from build123d import *

# Parameters (mm, degrees)
BOSS_EXTRUDE1_DEPTH = 6
CUT_EXTRUDE1_DEPTH  = 6


with BuildPart() as part:
    # Sketch1 → Boss-Extrude1 (new body)
    with BuildSketch(Plane.XY):
        with BuildLine():
            Line((20, 0), (260, 0))
            ThreePointArc((260, 0), (274.142135624, 5.857864376), (280, 20))
            Line((280, 20), (280, 140))
            ThreePointArc((280, 140), (274.142135624, 154.142135624), (260, 160))
            Line((260, 160), (20, 160))
            ThreePointArc((20, 160), (5.857864376, 154.142135624), (0, 140))
            Line((0, 140), (0, 20))
            ThreePointArc((0, 20), (5.857864376, 5.857864376), (20, 0))
        make_face()
    extrude(amount=BOSS_EXTRUDE1_DEPTH)

    # Sketch2 → Cut-Extrude1 (cut)
    with BuildSketch(Plane.XY.offset(6)):
        with BuildLine():
            Line((20, 137.5), (45, 137.5))
            Line((45, 137.5), (45, 122))
            ThreePointArc((45, 122), (47.784318939, 121.672513356), (50.416666667, 120.707928008))
            ThreePointArc((50.416666667, 120.707928008), (53.049014395, 121.672513356), (55.833333333, 122))
            Line((55.833333333, 122), (55.833333333, 137.5))
            Line((55.833333333, 137.5), (80.833333333, 137.5))
            Line((80.833333333, 137.5), (80.833333333, 122))
            ThreePointArc((80.833333333, 122), (83.617652272, 121.672513356), (86.25, 120.707928008))
            ThreePointArc((86.25, 120.707928008), (88.882347728, 121.672513356), (91.666666667, 122))
            Line((91.666666667, 122), (91.666666667, 137.5))
            Line((91.666666667, 137.5), (116.666666667, 137.5))
            Line((116.666666667, 137.5), (116.666666667, 122))
            ThreePointArc((116.666666667, 122), (119.450985605, 121.672513356), (122.083333333, 120.707928008))
            ThreePointArc((122.083333333, 120.707928008), (124.715681061, 121.672513356), (127.5, 122))
            Line((127.5, 122), (127.5, 137.5))
            Line((127.5, 137.5), (152.5, 137.5))
            Line((152.5, 137.5), (152.5, 122))
            ThreePointArc((152.5, 122), (155.284318939, 121.672513356), (157.916666667, 120.707928008))
            ThreePointArc((157.916666667, 120.707928008), (160.549014395, 121.672513356), (163.333333333, 122))
            Line((163.333333333, 122), (163.333333333, 137.5))
            Line((163.333333333, 137.5), (188.333333333, 137.5))
            Line((188.333333333, 137.5), (188.333333333, 122))
            ThreePointArc((188.333333333, 122), (191.117652272, 121.672513356), (193.75, 120.707928008))
            ThreePointArc((193.75, 120.707928008), (196.382347728, 121.672513356), (199.166666667, 122))
            Line((199.166666667, 122), (199.166666667, 137.5))
            Line((199.166666667, 137.5), (224.166666667, 137.5))
            Line((224.166666667, 137.5), (224.166666667, 122))
            ThreePointArc((224.166666667, 122), (226.950985605, 121.672513356), (229.583333333, 120.707928008))
            ThreePointArc((229.583333333, 120.707928008), (232.215681061, 121.672513356), (235, 122))
            Line((235, 122), (235, 137.5))
            Line((235, 137.5), (260, 137.5))
            Line((260, 137.5), (260, 122))
            ThreePointArc((260, 122), (272, 110), (260, 98))
            Line((260, 98), (260, 22.5))
            Line((260, 22.5), (235, 22.5))
            Line((235, 22.5), (235, 98))
            ThreePointArc((235, 98), (232.215681061, 98.327486644), (229.583333333, 99.292071992))
            ThreePointArc((229.583333333, 99.292071992), (226.950985605, 98.327486644), (224.166666667, 98))
            Line((224.166666667, 98), (224.166666667, 22.5))
            Line((224.166666667, 22.5), (199.166666667, 22.5))
            Line((199.166666667, 22.5), (199.166666667, 98))
            ThreePointArc((199.166666667, 98), (196.382347728, 98.327486644), (193.75, 99.292071992))
            ThreePointArc((193.75, 99.292071992), (191.117652272, 98.327486644), (188.333333333, 98))
            Line((188.333333333, 98), (188.333333333, 22.5))
            Line((188.333333333, 22.5), (163.333333333, 22.5))
            Line((163.333333333, 22.5), (163.333333333, 98))
            ThreePointArc((163.333333333, 98), (160.549014395, 98.327486644), (157.916666667, 99.292071992))
            ThreePointArc((157.916666667, 99.292071992), (155.284318939, 98.327486644), (152.5, 98))
            Line((152.5, 98), (152.5, 22.5))
            Line((152.5, 22.5), (127.5, 22.5))
            Line((127.5, 22.5), (127.5, 98))
            ThreePointArc((127.5, 98), (124.715681061, 98.327486644), (122.083333333, 99.292071992))
            ThreePointArc((122.083333333, 99.292071992), (119.450985605, 98.327486644), (116.666666667, 98))
            Line((116.666666667, 98), (116.666666667, 22.5))
            Line((116.666666667, 22.5), (91.666666667, 22.5))
            Line((91.666666667, 22.5), (91.666666667, 98))
            ThreePointArc((91.666666667, 98), (88.882347728, 98.327486644), (86.25, 99.292071992))
            ThreePointArc((86.25, 99.292071992), (83.617652272, 98.327486644), (80.833333333, 98))
            Line((80.833333333, 98), (80.833333333, 22.5))
            Line((80.833333333, 22.5), (55.833333333, 22.5))
            Line((55.833333333, 22.5), (55.833333333, 98))
            ThreePointArc((55.833333333, 98), (53.049014395, 98.327486644), (50.416666667, 99.292071992))
            ThreePointArc((50.416666667, 99.292071992), (47.784318939, 98.327486644), (45, 98))
            Line((45, 98), (45, 22.5))
            Line((45, 22.5), (20, 22.5))
            Line((20, 22.5), (20, 98))
            ThreePointArc((20, 98), (8, 110), (20, 122))
            Line((20, 122), (20, 137.5))
        make_face()
    extrude(amount=-CUT_EXTRUDE1_DEPTH, mode=Mode.SUBTRACT)


solid = part.part
Work out the finished part from the listing and answer in its coordinate system (mm). Coordinates: 2 decimals unless noted, no trailing zeros. Write each loop counter-clockwise with the first axis right and the second up, starting at its lowest first coordinate (ties: lowest second). Pieces come first, ordered by that corner, then holes. Notation, with made-up numbers: M 26,79.25 L 56,79.25 A14 ccw 56,90.25 Z; hole C -19.5,9.25 d10. An arc over 180 degrees is marked long. Write item = value, one per line.
1. Determine the mould class of faces 1 (the face through (6.014, 154.297, 2.958)), 2 (the face through (5.703, 6.014, 2.958)), 3 (the face through (88.92, 98.32, 3.04)) for opening direction Y: released by +Y, released by -Y, zero draft, split by the parting line, or undercut.
Solution:
face_1 = released by +Y
face_2 = released by -Y
face_3 = undercut
2. The part is cut by section B-B (y = 94.5). State how many separate pieces and enclosed holes the cut face has, then the cut area to 3 significant figures.
Solution:
separate_pieces = 8
enclosed_holes = 0
area = 630 mm2
3. Straight lines are drawn through the part: line 1 (Y direction, x = 214.5, z = 3.25); line 2 (Y direction, x = 224.5, z = 4.15); line 3 (X direction, y = 19.5, z = 0.5). For each, find the intervals that lie inside material, in ascending order. Write a range as from..to.
Solution:
line_1 = 0..22.5, 137.5..160
line_2 = 0..98, 122..160
line_3 = 0.01..279.99
4. The part is cut by section C-C (y = 11). Determine the outline of the cut face in (x, z).
Solution:
outline = M 2.14,0 L 277.86,0 L 277.86,6 L 2.14,6 Z
5. The part is cut by section A-A (x = 166.5). Determine the outline of the cut face in (y, z), then the cut area to 3 significant figures.
Solution:
outline = M 0,0 L 22.5,0 L 22.5,6 L 0,6 Z; M 137.5,0 L 160,0 L 160,6 L 137.5,6 Z
area = 270 mm2
